Geometry check sheet. Reference: the model listing, model coordinates, mm. A direction names the side the tool comes from. Give positions to 0.01 mm unless a question says otherwise; leave off trailing zeros. Write each loop counter-clockwise with the first axis right and the second up, starting at its lowest first coordinate (ties: lowest second). Pieces come first, ordered by that corner, then holes. Notation, with made-up numbers: (19, -13.5) - (76, -13.5) arc R14 cw to (76, -5.5) - close; hole circle Ø7 at (22.5, 15.5). An arc over 180 degrees is marked (long way). Use a Markdown table: item, result.
```python
from build123d import *

# Parameters (mm, degrees)
SKETCH1_W               = 45
SKETCH1_H               = 74
SKETCH1_R               = 5
BOSS_EXTRUDE1_DEPTH     = 2
SKETCH2_W               = 2
SKETCH2_H               = 74
BOSS_EXTRUDE2_DEPTH     = 23
SKETCH3_R               = 1.5
CUT_EXTRUDE1_DEPTH      = 44
CUT_EXTRUDE1_DEPTH_BACK = 3
FILLET1_R               = 20


with BuildPart() as part:
    # Sketch1 → Boss-Extrude1 (new body)
    with BuildSketch(Plane(origin=(0, 0, 0), x_dir=(1, 0, 0), z_dir=(0, 1, 0))):
        with Locations((-8, 0)):
            Rectangle(SKETCH1_W, SKETCH1_H)
        Circle(SKETCH1_R, mode=Mode.SUBTRACT)
    extrude(amount=BOSS_EXTRUDE1_DEPTH)

    # Sketch2 → Boss-Extrude2 (add)
    with BuildSketch(Plane(origin=(0, 2, 0), x_dir=(1, 0, 0), z_dir=(0, 1, 0))):
        with Locations((-29.5, 0)):
            Rectangle(SKETCH2_W, SKETCH2_H)
    extrude(amount=BOSS_EXTRUDE2_DEPTH)

    # Sketch3 → Cut-Extrude1 (cut, two sides)
    with BuildSketch(Plane(origin=(-28.5, 0, 0), x_dir=(0, 0, -1), z_dir=(1, 0, 0))) as cut_extrude1_sk:
        with Locations((-30, 18)):
            Circle(SKETCH3_R)
        with Locations((-30, 7)):
            Circle(SKETCH3_R)
        with Locations((30, 7)):
            Circle(SKETCH3_R)
        with Locations((30, 18)):
            Circle(SKETCH3_R)
    extrude(amount=CUT_EXTRUDE1_DEPTH, mode=Mode.SUBTRACT)
    extrude(cut_extrude1_sk.sketch, amount=-CUT_EXTRUDE1_DEPTH_BACK, mode=Mode.SUBTRACT)

    # Fillet1
    fillet1_edges = [part.edges().sort_by_distance(p)[0] for p in [
        (14.5, 1, -37),
        (14.5, 1, 37),
    ]]
    fillet(fillet1_edges, radius=FILLET1_R)


solid = part.part
```
1) Section check C-C on x = 4. Record the boundary of the cut face in (y, z).
Working result:
| item | result |
|---|---|
| outline | (0, -34.6) - (2, -34.6) - (2, -3) - (0, -3) - close; (0, 3) - (2, 3) - (2, 34.6) - (0, 34.6) - close |
2) Mould release check, pull along Z, two halves, no side actions. Record for faces 3 (the cylindrical face through (-29.49, 7.07, 31.5)), 4 (the cylindrical face through (-1.08, 0.99, 4.88)), 5 (the flat face through (-29, 7, 37)), 6 (the flat face through (-29, 7, -37)): pulls with the +Z half, pulls with the -Z half, needs draft (parallel to the pull), parting line crosses it, or undercut.
Working result:
| item | result |
|---|---|
| face 3 | undercut |
| face 4 | undercut |
| face 5 | pulls with the +Z half |
| face 6 | pulls with the -Z half |
3) Material ranges on L1, parallel to Y at x = -29, z = -30; L2, parallel to X at y = 10.75, z = 3; L3, parallel to Y at x = -10.5, z = 32.5, recorded low to high. Write a range as from..to.
Working result:
| item | result |
|---|---|
| L1 | y = 0..5.5, 8.5..16.5, 19.5..25 |
| L2 | x = -30.5..-28.5 |
| L3 | y = 0..2 |
4) Section check B-B on z = 0. Record the boundary of the cut face in (x, y).
Working result:
| item | result |
|---|---|
| outline | (-30.5, 0) - (-5, 0) - (-5, 2) - (-28.5, 2) - (-28.5, 25) - (-30.5, 25) - close; (5, 0) - (14.5, 0) - (14.5, 2) - (5, 2) - close |
5) Set-up check for faces 1 (the flat face through (-30.5, 12, 1)), 2 (the flat face through (-7, 2, -1)): record each of +Z, -Z, +X, -X, +Y, -Y from which the full face is reachable in a straight line by a thin tool's end or side.
Working result:
| item | result |
|---|---|
| face 1 | +Z, -Z, -X, +Y, -Y |
| face 2 | +Z, -Z, +X, +Y |
6) Section check D-D on z = -14. Record the boundary of the cut face in (x, y), then the cut area to 3 significant figures.
Working result:
| item | result |
|---|---|
| outline | (-30.5, 0) - (14.5, 0) - (14.5, 2) - (-28.5, 2) - (-28.5, 25) - (-30.5, 25) - close |
| area | 136 mm² |
7) Section check A-A on y = 7. Record the boundary of the cut face in (x, z), then the cut area to 3 significant figures.
Working result:
| item | result |
|---|---|
| outline | (-30.5, -37) - (-28.5, -37) - (-28.5, -31.5) - (-30.5, -31.5) - close; (-30.5, -28.5) - (-28.5, -28.5) - (-28.5, 28.5) - (-30.5, 28.5) - close; (-30.5, 31.5) - (-28.5, 31.5) - (-28.5, 37) - (-30.5, 37) - close |
| area | 136 mm² |
8) Depth check by flat-ended pin: P1, Ø13, axis at x = -2.5, z = -9.5, coming from the +Y side; P2, Ø6, axis at y = 10.5, z = -6.5, coming from the +X side. Enter the tip coordinate at first touch or a pass-through.
Working result:
| item | result |
|---|---|
| P1 | stops at y = 2 |
| P2 | stops at x = -28.5 |
